Could you check a few things on this model? Use its own coordinates, in mm. Face numbers are marked on the shaded views. A direction names the side the tool comes from. Coordinates: 2 decimals unless noted, no trailing zeros. Write each loop counter-clockwise with the first axis right and the second up, starting at its lowest first coordinate (ties: lowest second). Pieces come first, ordered by that corner, then holes. Notation, with made-up numbers: (73, 56) - (89, 56) arc R27 ccw to (89, 94) - close; hole circle Ø6 at (18.25, 56). An arc over 180 degrees is marked (long way). Answer as a JSON object with one key per item and string values. Group by question number.
1) If we section it at B-B (z = 6.5): Write out the boundary of the cut face in (x, y).
2) Please list where these lines run through material, in increasing order: line 1 along Z through (x, y) = (24, -26.5); line 2 along Z through (x, y) = (-22, -10); line 3 along X through (y, z) = (-19.75, 4.5).
3) If we section it at C-C (x = -43.5): Write out the boundary of the cut face in (y, z).
4) If we section it at D-D (x = -8.5): Write out the boundary of the cut face in (y, z).
5) Will these pins go through, and if not, where does the flat tip stop? pin 1 Ø8 at (y, z) = (-12, 4) entering from -X; pin 2 Ø5 at (x, y) = (49.5, -3) entering from -Z; pin 3 Ø14 at (x, y) = (-25.5, -18) entering from +Z.
6) We'd pull the mould along X, two halves only. Please class the marked faces 4, 5, 6 and 7: released by +X, released by -X, zero draft, split by the parting line, or undercut.
7) On a 3-axis mill with a long thin cutter (end or side, diameter ignored), from which of +Z, -Z, +X, -X, +Y, -Y can I reach the whole of each face in a straight line? I mean the marked faces 1, 2 and 3. Say none if no direction works.
8) If we section it at A-A (y = -16): Write out the boundary of the cut face in (x, z), plus the area to 3 significant figures.
```python
from build123d import *

# Parameters (mm, degrees)
F1_DEPTH = 28
F2_R     = 2
F3_R     = 1


with BuildPart() as f1:
    # F0 (on Front) → F1 (new body)
    with BuildSketch(Plane.XZ):
        Polygon((-51.000001, 2), (-51.000001, 0), (-10.433916, 0), (15.566084, 16), (62.999999, 16), (62.999999, 0), (64.999999, 0), (64.999999, 18), (14.999999, 18), (-11.000001, 2), align=None)
    extrude(amount=F1_DEPTH)

    # F2
    f2_edges = [f1.edges().sort_by_distance(p)[0] for p in [
        (14.999999, -14, 18),
        (64.999999, -14, 18),
        (-10.433916, -14, 0),
    ]]
    fillet(f2_edges, radius=F2_R)

    # F3
    f3_edges = [f1.edges().sort_by_distance(p)[0] for p in [
        (-11.000001, -14, 2),
        (62.999999, -14, 16),
        (15.566084, -14, 16),
    ]]
    fillet(f3_edges, radius=F3_R)


solid = f1.part
```
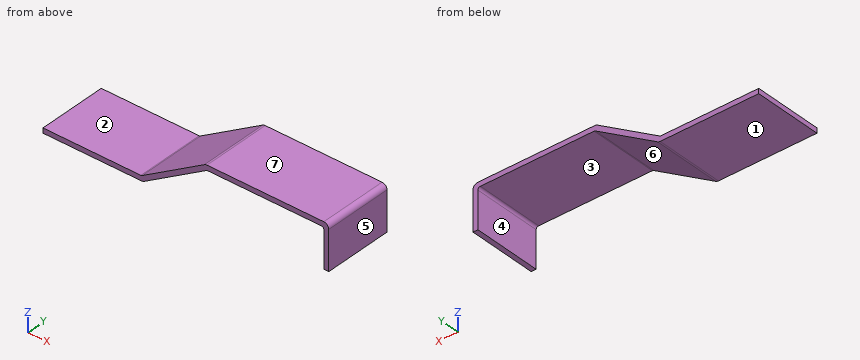
Here are the results:
{
 "1": {"outline": "(-3.69, -28) - (0.13, -28) - (0.13, 0) - (-3.69, 0) - close; (63, -28) - (65, -28) - (65, 0) - (63, 0) - close"},
 "2": {"line 1": "z = 16 to 18", "line 2": "z = 0 to 2", "line 3": "x = -6.94 to -3.12, 63 to 65"},
 "3": {"outline": "(-28, 0) - (0, 0) - (0, 2) - (-28, 2) - close"},
 "4": {"outline": "(-28, 1.19) - (0, 1.19) - (0, 3.54) - (-28, 3.54) - close"},
 "5": {"pin 1": "stops at x = -51", "pin 2": "stops at z = 16", "pin 3": "stops at z = 2"},
 "6": {"face 4": "undercut", "face 5": "released by +X", "face 6": "undercut", "face 7": "zero draft"},
 "7": {"face 1": "-Z, +X, -X, +Y, -Y", "face 2": "+Z, -X, +Y, -Y", "face 3": "-Z, +Y, -Y"},
 "8": {"outline": "(-51, 0) - (-11, 0) arc R2 ccw to (-9.95, 0.3) - (15.33, 15.85) arc R1 cw to (15.85, 16) - (62, 16) arc R1 cw to (63, 15) - (63, 0) - (65, 0) - (65, 16) arc R2 ccw to (63, 18) - (15.57, 18) arc R2 ccw to (14.52, 17.7) - (-10.76, 2.15) arc R1 cw to (-11.28, 2) - (-51, 2) - close", "area": "272 mm²"}
}
